```python
from build123d import *
from build123d.topology import SkipClean

# Parameters (mm, degrees)
BOSS_EXTRUDE1_DEPTH = 10


with BuildPart() as part:
    # Sketch1 → Boss-Extrude1 (new body)
    with BuildSketch(Plane(origin=(0, 0, 0), x_dir=(-1, 0, 0), z_dir=(0, 0, 1))):
        with BuildLine():
            Line((0, 0), (10.014962741, 0))
            ThreePointArc((10.014962741, 0), (28.514962741, 18.5), (47.014962741, 0))
            Line((47.014962741, 0), (118.514962741, 0))
            ThreePointArc((118.514962741, 0), (128.514962741, 10), (138.514962741, 0))
            Line((138.514962741, 0), (158.514962741, 0))
            ThreePointArc((158.514962741, 0), (168.514962741, 10), (178.514962741, 0))
            Line((178.514962741, 0), (188.514962741, 0))
            ThreePointArc((188.514962741, 0), (183.080821195, 13.70531895), (169.73138599, 19.962973588))
            Line((169.73138599, 19.962973588), (30.249275922, 28.462172403))
            ThreePointArc((30.249275922, 28.462172403), (8.974629781, 20.767245555), (0, 0))
        make_face()
    boss_extrude1 = extrude(amount=BOSS_EXTRUDE1_DEPTH)

    # Mirror1: Boss-Extrude1 across plane
    with SkipClean():  # the faces are left unmerged after this step: merging them gives an invalid solid
        add(boss_extrude1.mirror(Plane(origin=(-47.014962741, 0, 10), x_dir=(0, 0, 1), z_dir=(0, -1, 0))))


solid = part.part
```
Here's how the part is built. I have some questions about the finished solid (model axes, mm). Round coordinates to 2 decimals unless told otherwise and drop trailing zeros. Order: outer loops, then holes, each group sorted by start corner. A loop starts at its lowest first (then second) coordinate and runs counter-clockwise, first axis right, second up. Notation, with made-up numbers: M 19.5,-18 L 55.5,-18 A27 cw 55.5,14 Z; hole C -40,-24 d5. An arc over 180 degrees is marked long. Answer in a Markdown table with one row per item.
Item 1: Thinking about a two-plate mould opening in X: for faces 1 (the face through (-100.967, 24.153, 4.93)), 2 (the face through (-159.278, -3.83, 4.93)), 3 (the face through (-93, 0, 10)), which applies, +X half, -X half, draft (parallel to the pull), parting line (faces both ways), or undercut?
A:
| item | result |
|---|---|
| face 1 | -X half |
| face 2 | undercut |
| face 3 | draft |
Item 2: Imagine slicing it at B-B, the plane x = -125. Write out the boundary of the cut face in (y, z).
A:
| item | result |
|---|---|
| outline | M -22.69,0 L -9.36,0 L -9.36,10 L -22.69,10 Z; M 9.36,0 L 22.69,0 L 22.69,10 L 9.36,10 Z |
Item 3: Imagine slicing it at C-C, the plane y = 7. Write out the boundary of the cut face in (x, z), and give its area (3 significant figures).
A:
| item | result |
|---|---|
| outline | M -187.25,0 L -175.66,0 L -175.66,10 L -187.25,10 Z; M -161.37,0 L -135.66,0 L -135.66,10 L -161.37,10 Z; M -121.37,0 L -45.64,0 L -45.64,10 L -121.37,10 Z; M -11.39,0 L -0.87,0 L -0.87,10 L -11.39,10 Z |
| area | 1,240 mm2 |
Item 4: Imagine slicing it at D-D, the plane y = 15.5. Write out the boundary of the cut face in (x, z), and give its area (3 significant figures).
A:
| item | result |
|---|---|
| outline | M -181.15,0 L -38.61,0 L -38.61,10 L -181.15,10 Z; M -18.42,0 L -4.58,0 L -4.58,10 L -18.42,10 Z |
| area | 1,560 mm2 |
Item 5: If I drill on L1, parallel to X at y = 1, z = 1.5; L2, parallel to X at y = 0, z = 7.75; L3, parallel to Y at x = -40.5, z = 3, over which ranges is the centre line in solid material (lowest first)? Write a range as from..to.
A:
| item | result |
|---|---|
| L1 | x = -188.49..-178.46, -158.57..-138.46, -118.57..-46.99, -10.04..-0.02 |
| L2 | x = -188.51..-178.51, -158.51..-138.51, -118.51..-47.01, -10.01..0 |
| L3 | y = -27.84..-14.09, 14.09..27.84 |
Item 6: I'm going to push flat-ended pins straight in: pin 1 (5 mm diameter, centred on y = -17.5, z = 2.5, fed in from -X); pin 2 (2 mm diameter, centred on y = 5, z = 3, fed in from -X); pin 3 (5 mm diameter, centred on x = -109, z = 7, fed in from -Y). Where does each tip first touch, or does it pass through?
A:
| item | result |
|---|---|
| pin 1 | stops at x = -181.74 |
| pin 2 | stops at x = -188.11 |
| pin 3 | stops at y = -23.82 |
Item 7: Imagine slicing it at A-A, the plane z = 6.75. Write out the boundary of the cut face in (x, y).
A:
| item | result |
|---|---|
| outline | M -169.73,-19.96 L -30.25,-28.46 A28.51 ccw long -30.25,28.46 L -169.73,19.96 A20 ccw Z; hole C -168.51,0 d20; hole C -128.51,0 d20; hole C -28.51,0 d37 |
